Here's how the part is built. I have some questions about the finished solid (model axes, mm). A direction names the side the tool comes from. Round coordinates to 2 decimals unless told otherwise and drop trailing zeros. Write each loop counter-clockwise with the first axis right and the second up, starting at its lowest first coordinate (ties: lowest second). Pieces come first, ordered by that corner, then holes. Notation, with made-up numbers: (15.5, 6) - (27.5, 6) arc R23 ccw to (27.5, 45) - close; hole circle Ø3 at (-35, 72.25). An arc over 180 degrees is marked (long way). Use one line per item in the form item = value. Start each with the question number.
1. Will these pins go through, and if not, where does the flat tip stop? pin 1 (2 mm diameter, centred on y = -3.5, z = 1, fed in from -X); pin 2 (3 mm diameter, centred on y = -6.5, z = 3, fed in from +X).
2. I want a section at B-B, the plane y = 16. List the corners of the cut face in (x, z) for me.
3. We'd pull the mould along Y, two halves only. Please class faces 1 (the flat face through (-1, -25.4, 3)), 2 (the flat face through (-95.25, 6, 3)), 3 (the flat face through (-92, 0, 3)), 4 (the flat face through (-92, 12.7, 3)): +Y half, -Y half, draft (parallel to the pull), parting line (faces both ways), or undercut.
4. I want a section at A-A, the plane z = 2.75. List the corners of the cut face in (x, y) for me.
5. Which directions (+Z, -Z, +X, -X, +Y, -Y) give clear straight access to the entire face, cutting with the end or side of a thin tool? Please do faces 5 (the flat face through (-92, -12.7, 3)), 6 (the flat face through (92, 12.7, 3)), 7 (the flat face through (92, -12.7, 3)).
6. If I drill on line 1 along X through (y, z) = (-4, 2.25), over which ranges is the centre line in solid material (lowest first)?
```python
from build123d import *

# Parameters (mm, degrees)
SKETCH1_W               = 190.5
SKETCH1_H               = 50.8
BOSS_EXTRUDE1_DEPTH     = 6.35
SKETCH2_W               = 6.35
SKETCH2_H               = 12.7
CUT_EXTRUDE1_DEPTH      = 7.35
LPATTERN1_COUNT         = 2
LPATTERN1_PITCH         = 25.4
MIRROR1_COPY_1_SKETCH_W = 6.35
MIRROR1_COPY_1_SKETCH_H = 12.7
MIRROR1_COPY_1_DEPTH    = 7.35


with BuildPart() as part:
    # Sketch1 → Boss-Extrude1 (new body)
    with BuildSketch(Plane.XY):
        Rectangle(SKETCH1_W, SKETCH1_H)
    extrude(amount=BOSS_EXTRUDE1_DEPTH)

    # Sketch2 → Cut-Extrude1 (cut, through all)
    with BuildSketch(Plane.XY.offset(6.35)):
        with Locations((92.075, -6.35)):
            Rectangle(SKETCH2_W, SKETCH2_H)
    cut_extrude1 = extrude(amount=-CUT_EXTRUDE1_DEPTH, mode=Mode.SUBTRACT)

    # LPattern1: Cut-Extrude1 ×2
    with Locations(*[(0, i * LPATTERN1_PITCH, 0) for i in range(1, LPATTERN1_COUNT)]):
        add(cut_extrude1, mode=Mode.SUBTRACT)

    # Mirror1: Cut-Extrude1 across plane
    add(cut_extrude1.mirror(Plane(origin=(0, 0, 0), x_dir=(0, 0, 1), z_dir=(1, 0, 0))), mode=Mode.SUBTRACT)

    # Mirror1 copy 1 sketch → Mirror1 copy 1 (cut, through all)
    with BuildSketch(Plane(origin=(0, 25.4, 6.35), x_dir=(-1, 0, 0), z_dir=(0, 0, 1))):
        with Locations((92.075, 6.35)):
            Rectangle(MIRROR1_COPY_1_SKETCH_W, MIRROR1_COPY_1_SKETCH_H)
    extrude(amount=-MIRROR1_COPY_1_DEPTH, mode=Mode.SUBTRACT)


solid = part.part
```
Model answer:
q1.pin_1 = -88.9
q1.pin_2 = 88.9
q2.outline = (-88.9, 0) - (88.9, 0) - (88.9, 6.35) - (-88.9, 6.35) - close
q3.face_1 = -Y half
q3.face_2 = draft
q3.face_3 = undercut
q3.face_4 = +Y half
q4.outline = (-95.25, -25.4) - (95.25, -25.4) - (95.25, -12.7) - (88.9, -12.7) - (88.9, 0) - (95.25, 0) - (95.25, 12.7) - (88.9, 12.7) - (88.9, 25.4) - (-88.9, 25.4) - (-88.9, 12.7) - (-95.25, 12.7) - (-95.25, 0) - (-88.9, 0) - (-88.9, -12.7) - (-95.25, -12.7) - close
q5.face_5 = +Z, -Z, -X
q5.face_6 = +Z, -Z, +X, +Y
q5.face_7 = +Z, -Z, +X
q6.line_1 = -88.9 to 88.9
